Read the model definition and answer for the solid it produces. Units are mm, in the model's axes. Give positions to 0.01 mm unless a question says otherwise; leave off trailing zeros. Write each loop counter-clockwise with the first axis right and the second up, starting at its lowest first coordinate (ties: lowest second). Pieces come first, ordered by that corner, then holes. Notation, with made-up numbers: (45.5, -39.5) - (74.5, -39.5) arc R24 ccw to (74.5, -5.5) - close; hole circle Ø9 at (23, -21.75). An arc over 180 degrees is marked (long way). Answer as a JSON object with one key per item and string values. Group by question number.
Autodesk Inventor part; units mm, degrees
ref_plane "Work Plane6" through (38.1, 25.4, 0) normal (-0.4902612, 0.8715755, 0) x (0, 0, 1)
ref_plane "YZ Plane" through (0, 0, 0) normal (1, 0, 0) x (0, 1, 0)
ref_plane "XZ Plane" through (0, 0, 0) normal (0, 1, 0) x (-1, 0, 0)
sketch "Sketch1" plane through (0, 0, 0) normal (0, 0, 1) x (1, 0, 0)
  line L0 (0, 0) -> (12.7, 0)
  line L1 (12.7, 0) -> (38.1, 25.4)
  line L2 (38.1, 25.4) -> (38.1, 38.1)
  arc A0 (50.8, 50.8) -> (38.1, 38.1) centre (50.8, 38.1) ccw
  line L3 (0, 0) -> (0, 76.2)
  line L4 (0, 76.2) -> (19.05, 76.2)
  line L5 (19.05, 190.5) -> (19.05, 76.2)
  line L6 (38.1, 171.45) -> (38.1, 88.9)
  arc A1 (50.8, 50.8) -> (50.8, 76.2) centre (50.8, 63.5) ccw
  arc A2 (38.1, 88.9) -> (50.8, 76.2) centre (50.8, 88.9) ccw
  line L7 (19.05, 190.5) -> (101.6, 190.5)
  line L8 (82.55, 171.45) -> (38.1, 171.45)
  line L9 (101.6, 190.5) -> (101.6, 146.05)
  line L10 (101.6, 146.05) -> (82.55, 146.05)
  line L11 (82.55, 146.05) -> (82.55, 171.45)
  dimension "d1" = 25.4
  dimension "d2" = 25.4
  dimension "d3" = 12.7
  dimension "d38" = 76.2
  dimension "d41" = 38.1
  dimension "d84" = 12.7
  dimension "d85" = 12.7
  dimension "d87" = 0
  dimension "d88" = 12.7
  dimension "d90" = 19.05
  dimension "d100" = 19.05
  dimension "d101" = 19.05
  dimension "d102" = 19.05
  dimension "d103" = 107.95
  dimension "d104" = 44.45
  dimension "d105" = 25.4
extrude "Extrusion1" add sketch "Sketch1" along normal blind 9.525
sketch "Sketch3" plane through (0, 0, 9.525) normal (0, 0, 1) x (1, 0, 0)
  line L0 (0, 76.2) -> (0, 0)
  line L1 (0, 0) -> (12.7, 0)
  arc A0 (50.8, 50.8) -> (38.1, 38.1) centre (50.8, 38.1) ccw
  line L2 (19.05, 76.2) -> (0, 76.2)
  point P0 (50.8, 63.5)
  point P1 (49.53, 54.61)
  point P2 (12.7, 82.55)
  dimension "d39" = 0
  dimension "d40" = 12.7
hole "Hole2" at (50.8, 63.5, 9.525) direction (0, 0, -1) diameter 6.35 end through all
sketch "Sketch7" plane through (0, 76.2, 0) normal (0, 1, 0) x (1, 0, 0)
  line L0 (0, 0) -> (0, -9.525)
  point P0 (9.525, -4.7625)
  dimension "d77" = 9.525
ref_plane "Work Plane6" through (38.1, 25.4, 0) normal (-0.4902612, 0.8715755, 0) x (0, 0, 1)
ref_plane "Work Plane5" through (38.1, 25.4, 4.7625) normal (0.8715755, 0.4902612, 0) x (-0.4902612, 0.8715755, 0)
sketch "Sketch8" plane through (38.1, 25.4, 0) normal (-0.4902612, 0.8715755, 0) x (0, 0, 1)
  line L0 (0, 0) -> (9.525, 0)
  circle A0 centre (4.7625, 0) radius 2.7813
  point P0 (0, -45.6597)
  dimension "d79" = 5.5626
extrude "Extrusion3" cut sketch "Sketch8" along normal through all both and the other way through all
sketch "Sketch10" plane through (0, 0, 9.525) normal (0, 0, 1) x (1, 0, 0)
  circle A0 centre (50.8, 63.5) radius 3.175
  line L0 (0, 0) -> (12.7, 0)
  line L1 (12.7, 0) -> (38.1, 25.4)
  line L2 (38.1, 25.4) -> (38.1, 38.1)
  arc A1 (50.8, 50.8) -> (38.1, 38.1) centre (50.8, 38.1) ccw
  arc A2 (50.8, 50.8) -> (50.8, 76.2) centre (50.8, 63.5) ccw
  arc A3 (38.1, 88.9) -> (50.8, 76.2) centre (50.8, 88.9) ccw
  line L3 (38.1, 88.9) -> (38.1, 171.45)
  line L4 (19.05, 190.5) -> (19.05, 76.2)
  line L5 (19.05, 76.2) -> (0, 76.2)
  line L6 (0, 76.2) -> (0, 0)
  line L7 (12.7, 0) -> (38.1, 25.4)
  line L8 (31.75, 19.05) -> (0, 19.05)
  line L9 (38.1, 171.45) -> (82.55, 171.45)
  line L10 (82.55, 171.45) -> (82.55, 146.05)
  line L11 (82.55, 146.05) -> (101.6, 146.05)
  line L12 (101.6, 146.05) -> (101.6, 190.5)
  line L13 (101.6, 190.5) -> (19.05, 190.5)
  dimension "d95" = 6.35
extrude "Extrusion5" cut sketch "Sketch10" against normal through all contours L6 L8 L1 L0
fillet "Fillet6" radius 6.35 9 edges at (0, 76.2, 4.7625) (0, 19.05, 4.7625) (31.75, 19.05, 4.7625) (38.1, 25.4, 8.5344) (38.1, 25.4, 0.9906) (19.05, 190.5, 4.7625) (101.6, 190.5, 4.7625) (82.55, 146.05, 4.7625) (101.6, 146.05, 4.7625)
properties part number "CLB_079_ScissorHookV2"
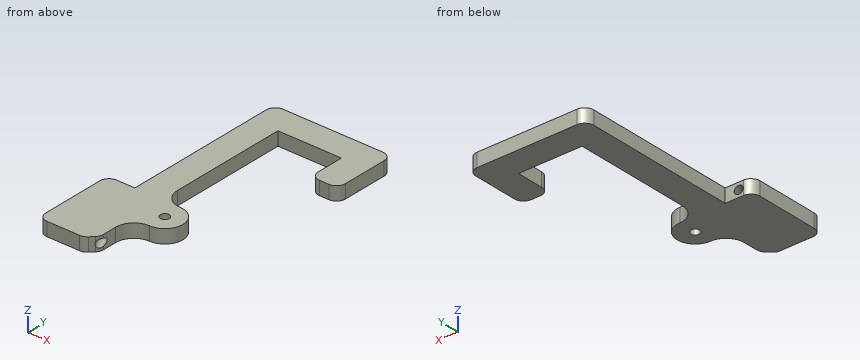
1) Flat-ended cylindrical pins translate along their axes: pin 1 Ø3 at (y, z) = (34.5, 5) entering from +X; pin 2 Ø5 at (y, z) = (165, 4.5) entering from -X. Find the tip coordinate at first contact, or state that the pin passes through.
2) Find section A-A, the plane y = 63.5. Give the number of separate pieces and of enclosed holes in the cut face, and give its area (3 significant figures).
3) Find the intervals of material crossed by line 1 (Y direction, x = 50.8, z = 6.5) (3 decimals); line 2 (X direction, y = 160.5, z = 8); line 3 (Y direction, x = 52, z = 3.75), in increasing order. Write a range as [from, to].
4) Find section C-C, the plane y = 106. Write down the section's boundary in (x, z) (3 decimals).
5) Find section B-B, the plane x = 76. Write down the section's boundary in (y, z) (3 decimals).
Values follow:
{
 "1": {"pin 1": "stops at x = 38.1", "pin 2": "stops at x = 19.05"},
 "2": {"separate pieces": "2", "enclosed holes": "1", "area": "516 mm2"},
 "3": {"line 1": "y = [50.8, 60.325], [66.675, 76.2], [171.45, 190.5]", "line 2": "x = [19.05, 38.1], [82.55, 101.6]", "line 3": "y = [50.86, 60.56], [66.44, 76.14], [171.45, 190.5]"},
 "4": {"outline": "(19.05, 0) - (38.1, 0) - (38.1, 9.525) - (19.05, 9.525) - close"},
 "5": {"outline": "(171.45, 0) - (190.5, 0) - (190.5, 9.525) - (171.45, 9.525) - close"}
}
